Read the model definition and answer for the solid it produces. Units are mm, in the model's axes. A direction names the side the tool comes from. Round coordinates to 2 decimals unless told otherwise and drop trailing zeros. Write each loop counter-clockwise with the first axis right and the second up, starting at its lowest first coordinate (ties: lowest second). Pieces come first, ordered by that corner, then holes. Notation, with made-up numbers: M 30,-13 L 75,-13 A19 ccw 75,-3 Z; hole C -20.75,-37.5 d9. An arc over 180 degrees is marked long. Use one line per item in the form item = value. Start each with the question number.
```python
from build123d import *

# Parameters (mm, degrees)
SKETCH_R        = 4.15
EXTRUDE_DEPTH   = 7
SKETCH001_R     = 1.55
POCKET_DEPTH    = 4
SKETCH002_R     = 2
POCKET001_DEPTH = 27.5798157383
POCKET002_DEPTH = 3.5
POCKET003_DEPTH = 2.25
POCKET004_DEPTH = 2.6


with BuildPart() as part:
    # Sketch → Extrude (new body)
    with BuildSketch(Plane.XY):
        with BuildLine():
            ThreePointArc((4.5, -13.6788157382), (0, 14.4), (-4.5, -13.6788157382))
            Line((-4.5, -13.6788157382), (-4.5, -17.1788157382))
            Line((-4.5, -17.1788157382), (4.5, -17.1788157382))
            Line((4.5, -17.1788157382), (4.5, -13.6788157382))
        make_face()
        Circle(SKETCH_R, mode=Mode.SUBTRACT)
        with BuildLine():
            ThreePointArc((-4.1103420039, 6.4519445605), (-7.65, 0), (-4.1103420039, -6.4519445605))
            ThreePointArc((-5.856565731, -9.1929667594), (-3.612942768, -8.6955675235), (-4.1103420039, -6.4519445605))
            ThreePointArc((-5.856565731, 9.1929667594), (-10.9, 0), (-5.856565731, -9.1929667594))
            ThreePointArc((-4.1103420039, 6.4519445605), (-3.612942768, 8.6955675235), (-5.856565731, 9.1929667594))
        make_face(mode=Mode.SUBTRACT)
        with BuildLine():
            ThreePointArc((4.1103420039, -6.4519445605), (7.65, 0), (4.1103420039, 6.4519445605))
            ThreePointArc((5.856565731, 9.1929667594), (3.612942768, 8.6955675235), (4.1103420039, 6.4519445605))
            ThreePointArc((5.856565731, -9.1929667594), (10.9, 0), (5.856565731, 9.1929667594))
            ThreePointArc((4.1103420039, -6.4519445605), (3.612942768, -8.6955675235), (5.856565731, -9.1929667594))
        make_face(mode=Mode.SUBTRACT)
    extrude(amount=EXTRUDE_DEPTH)

    # Sketch001 → Pocket (cut)
    with BuildSketch(Plane.XZ.offset(17.1788157382)):
        with Locations((0, 3.5)):
            Circle(SKETCH001_R)
    extrude(amount=-POCKET_DEPTH, mode=Mode.SUBTRACT)

    # Sketch002 → Pocket001 (cut, through all)
    with BuildSketch(Plane.XZ.offset(13.1788157382)):
        with Locations((0, 3.5)):
            Circle(SKETCH002_R)
    extrude(amount=-POCKET001_DEPTH, mode=Mode.SUBTRACT)

    # Sketch003 → Pocket002 (cut)
    with BuildSketch(Plane.XY.offset(7)):
        Polygon((1.55, -17.1788157382), (-1.55, -17.1788157382), (-1.55, -13.1788157382), (-3.125, -13.1788157382), (-3.125, -10.9288157382), (3.125, -10.9288157382), (3.125, -13.1788157382), (1.55, -13.1788157382), align=None)
    extrude(amount=-POCKET002_DEPTH, mode=Mode.SUBTRACT)

    # Sketch004 → Pocket003 (cut)
    with BuildSketch(Plane.XZ.offset(10.9288157382)):
        with BuildLine():
            Line((-3.125, 3.5), (3.125, 3.5))
            ThreePointArc((-3.125, 3.5), (0, 0.375), (3.125, 3.5))
        make_face()
    extrude(amount=POCKET003_DEPTH, mode=Mode.SUBTRACT)

    # Sketch005 → Pocket004 (cut)
    with BuildSketch(Plane.XY.offset(7)):
        with BuildLine():
            ThreePointArc((-3.3043925913, 5.1868573917), (-2.3478555993, 9.501516936), (-6.6625151435, 10.4580539281))
            ThreePointArc((-6.6625151435, 10.4580539281), (-12.4, 0), (-6.6625151435, -10.4580539281))
            ThreePointArc((-6.6625151435, -10.4580539281), (-2.3478555993, -9.501516936), (-3.3043925913, -5.1868573918))
            ThreePointArc((-3.3043925913, 5.1868573917), (-6.15, 0), (-3.3043925913, -5.1868573918))
        make_face()
        with BuildLine():
            ThreePointArc((6.6625151435, 10.4580539281), (2.3478555993, 9.501516936), (3.3043925913, 5.1868573917))
            ThreePointArc((3.3043925913, -5.1868573917), (6.15, 0), (3.3043925913, 5.1868573917))
            ThreePointArc((3.3043925913, -5.1868573917), (2.3478555993, -9.501516936), (6.6625151435, -10.4580539281))
            ThreePointArc((6.6625151435, -10.4580539281), (12.4, 0), (6.6625151435, 10.4580539281))
        make_face()
    extrude(amount=-POCKET004_DEPTH, mode=Mode.SUBTRACT)


solid = part.part
```
Q1. For a pull along Y with two mould halves and no side action, classify faces 5 (the face through (6.15, -0.09, 5.72)), 6 (the face through (1.908, -7.334, 4.101)), 7 (the face through (-3.632, -8.725, 2.169)), 8 (the face through (-1, -17.179, 2)) as +Y half, -Y half, draft (parallel to the pull), parting line (faces both ways), or undercut.
Q2. Straight lines are drawn through the part: line 1 (X direction, y = -7, z = 4); line 2 (Z direction, x = 0, y = 7.5); line 3 (Y direction, x = 3.5, z = 5.75). For each, find the intervals that lie inside material, in ascending order. Write a range as [from, to].
Q3. Each of these flat-tipped pins is pushed along its axis until it touches: pin 1 Ø3 at (x, z) = (0, 3.5) entering from -Y; pin 2 Ø1.8 at (y, z) = (-16, 2.5) entering from +X; pin 3 Ø4 at (y, z) = (-16, 5) entering from -X; pin 4 Ø0.7 at (y, z) = (-12, 5.5) entering from -X. Where does it stop, or does it pass through?
Q4. A tool of negligible diameter and unlimited length cuts with its end or side. For faces 1 (the face through (-4.5, -15, 3)), 2 (the face through (-2.385, -9.559, 5.718)), 3 (the face through (-1.55, -15, 5)), 4 (the face through (-3.594, 8.665, 2.169)), from which of +Z, -Z, +X, -X, +Y, -Y can it reach the whole face along a straight path? Write none if from no direction.
Q5. Find section C-C on x = 0. Write down the section's boundary in (y, z) (3 decimals), and give its area (3 significant figures).
Q6. Find section A-A on z = 4. Count the separate pieces of the cut face and the enclosed holes in it, and give its area (3 significant figures).
Q7. Find section B-B on y = 0. Write down the section's boundary in (x, z), and give its area (3 significant figures).
Q8. Find section D-D on z = 6.5. Write down the section's boundary in (x, y) (3 decimals), and give its area (3 significant figures).
Response:
q1.face_5 = undercut
q1.face_6 = draft
q1.face_7 = undercut
q1.face_8 = -Y half
q2.line_1 = [-12.58, -8.36], [-3.58, -1.94], [1.94, 3.58], [8.36, 12.58]
q2.line_2 = [0, 1.5], [5.5, 7]
q2.line_3 = [-17.18, -10.57], [-5.06, -2.23], [2.23, 5.06], [10.57, 13.97]
q3.pin_1 = through
q3.pin_2 = 4.5
q3.pin_3 = -4.5
q3.pin_4 = -8.46
q4.face_1 = +Z, -Z, -X, -Y
q4.face_2 = +Z
q4.face_3 = +Z, -Y
q4.face_4 = +Z, -Z
q5.outline = M -17.179,0 L -4.15,0 L -4.15,1.5 L -10.929,1.5 L -10.929,0.375 L -13.179,0.375 L -13.179,1.95 L -17.179,1.95 Z; M -10.929,5.5 L -4.15,5.5 L -4.15,7 L -10.929,7 Z; M 4.15,0 L 14.4,0 L 14.4,1.5 L 4.15,1.5 Z; M 4.15,5.5 L 14.4,5.5 L 14.4,7 L 4.15,7 Z
q5.area = 59.7 mm²
q6.separate_pieces = 2
q6.enclosed_holes = 2
q6.area = 393 mm²
q7.outline = M -14.4,0 L -10.9,0 L -10.9,4.4 L -12.4,4.4 L -12.4,7 L -14.4,7 Z; M -7.65,0 L -4.15,0 L -4.15,7 L -6.15,7 L -6.15,4.4 L -7.65,4.4 Z; M 4.15,0 L 7.65,0 L 7.65,4.4 L 6.15,4.4 L 6.15,7 L 4.15,7 Z; M 10.9,0 L 14.4,0 L 14.4,7 L 12.4,7 L 12.4,4.4 L 10.9,4.4 Z
q7.area = 82.4 mm²
q8.outline = M -4.5,-17.179 L -1.55,-17.179 L -1.55,-13.179 L -3.125,-13.179 L -3.125,-10.929 L 3.125,-10.929 L 3.125,-13.179 L 1.55,-13.179 L 1.55,-17.179 L 4.5,-17.179 L 4.5,-13.679 A14.4 ccw long -4.5,-13.679 Z; hole M -6.663,-10.458 A3.125 ccw -3.304,-5.187 A6.15 cw -3.304,5.187 A3.125 ccw -6.663,10.458 A12.4 ccw Z; hole C 0,0 d8.3; hole M 3.304,-5.187 A3.125 ccw 6.663,-10.458 A12.4 ccw 6.663,10.458 A3.125 ccw 3.304,5.187 A6.15 cw Z
q8.area = 304 mm²
